Input: part model. Units: mm. Frame: model coordinates. Face numbers are marked on the shaded views. A direction names the side the tool comes from. Give positions to 0.01 mm unless a question says otherwise; leave off trailing zeros. Loops run counter-clockwise (first coordinate to the right, second up) from the corner with the lowest first, then second, coordinate; pieces in that order, holes last. Notation, with made-up numbers: (83, 77) -> (117, 77) arc R36 ccw to (117, 116) -> close; hole circle Ø8 at (22.25, 42). An arc over 180 degrees is marked (long way). One line per question, with ' | ' between items.
from build123d import *

# Parameters (mm, degrees)
SZKIC1_R                    = 323.75
DODANIE_WYCI_GNI_CIE1_DEPTH = 381
ZAOKR_GLENIE1_R             = 50
SZKIC2_R                    = 6.5
SZKIC2_R_2                  = 30
WYTNIJ_WYCI_GNI_CIE1_DEPTH  = 596.641775734
SZKIC3_R                    = 250
WYTNIJ_WYCI_GNI_CIE2_DEPTH  = 50
WYTNIJ_WYCI_GNI_CIE3_START  = -200
SZKIC4_R                    = 250
WYTNIJ_WYCI_GNI_CIE3_DEPTH  = 200
WYTNIJ_WYCI_GNI_CIE4_DEPTH  = 200
WYTNIJ_WYCI_GNI_CIE5_START  = -80
SZKIC6_R                    = 250
SZKIC6_R_2                  = 85
WYTNIJ_WYCI_GNI_CIE5_DEPTH  = 80


with BuildPart() as part:
    # Szkic1 → Dodanie-wyciągnięcie1 (new body)
    with BuildSketch(Plane.XY):
        Circle(SZKIC1_R)
    extrude(amount=DODANIE_WYCI_GNI_CIE1_DEPTH)

    # Zaokrąglenie1
    zaokr_glenie1_edges = [part.edges().sort_by_distance(p)[0] for p in [
        (-323.75, 0, 0),
        (-323.75, 0, 381),
    ]]
    fillet(zaokr_glenie1_edges, radius=ZAOKR_GLENIE1_R)

    # Szkic2 → Wytnij-wyciągnięcie1 (cut, through all)
    with BuildSketch(Plane.XY.offset(381)):
        with Locations((-60, 0)):
            Circle(SZKIC2_R)
        with Locations((-18.541019662, 57.063390978)):
            Circle(SZKIC2_R)
        with Locations((48.541019662, 35.267115138)):
            Circle(SZKIC2_R)
        with Locations((48.541019662, -35.267115138)):
            Circle(SZKIC2_R)
        with Locations((-18.541019662, -57.063390978)):
            Circle(SZKIC2_R)
        Circle(SZKIC2_R_2)
    extrude(amount=-WYTNIJ_WYCI_GNI_CIE1_DEPTH, mode=Mode.SUBTRACT)

    # Szkic3 → Wytnij-wyciągnięcie2 (cut)
    with BuildSketch(Plane.XY.offset(381)):
        Circle(SZKIC3_R)
    extrude(amount=-WYTNIJ_WYCI_GNI_CIE2_DEPTH, mode=Mode.SUBTRACT)

    # Szkic4 → Wytnij-wyciągnięcie3 (cut)
    with BuildSketch(Plane(origin=(0, 0, 0), x_dir=(-1, 0, 0), z_dir=(0, 0, -1)).offset(WYTNIJ_WYCI_GNI_CIE3_START)):
        with Locations(Location((0, 0, 0), (0, 0, 180))):
            Circle(SZKIC4_R)
    extrude(amount=WYTNIJ_WYCI_GNI_CIE3_DEPTH, mode=Mode.SUBTRACT)

    # Szkic5 → Wytnij-wyciągnięcie4 (cut)
    with BuildSketch(Plane.XY.offset(331)):
        Polygon((-96.155840105, 0), (-149.925673453, 63.746040452), (-231.191444309, 44.19337378), (-220.558452121, 0), (-96.155840105, -44.404647078), align=None)
        Polygon((-102.20240394, 27.791849476), (-73.659646986, 61.807782618), (-73.87456406, 145.202665329), (-148.695968113, 182.461084274), (-168.95757663, 141.772240235), align=None)
        Polygon((-60.427327118, 86.984230788), (-16.697286406, 94.695016833), (36.743274881, 158.71734935), (3.376004134, 235.353225607), (-38.29957328, 217.207673641), align=None)
        Polygon((9.622367637, 105.475723792), (48.077920052, 83.273400253), (130.168527149, 97.966421664), (153.868306527, 178.120977019), (110.279226061, 191.009222556), align=None)
        Polygon((75.169649634, 74.613953402), (90.356933392, 32.887234214), (162.686478902, -8.624083495), (232.36391824, 37.543943689), (207.25714991, 75.435433406), align=None)
        Polygon((105.54421715, 8.839484973), (90.356933392, -32.887234214), (119.081619118, -111.17928414), (202.133870171, -120.600318147), (207.25714991, -75.435433406), align=None)
        Polygon((86.533472468, -61.071076714), (48.077920052, -83.273400253), (19.757146304, -161.712462116), (77.323137782, -222.314350799), (110.279226061, -191.009222556), align=None)
        Polygon((27.032754306, -102.405802878), (-16.697286406, -94.695016833), (-88.811914842, -136.578581834), (-83.667950127, -220.005027963), (-38.29957328, -217.207673641), align=None)
        Polygon((-45.116890032, -95.823715761), (-73.659646986, -61.807782618), (-155.824893999, -47.53806521), (-205.509874305, -114.75290746), (-168.95757663, -141.772240235), align=None)
    extrude(amount=-WYTNIJ_WYCI_GNI_CIE4_DEPTH, mode=Mode.SUBTRACT)

    # Szkic6 → Wytnij-wyciągnięcie5 (cut)
    with BuildSketch(Plane(origin=(0, 0, 200), x_dir=(-1, 0, 0), z_dir=(0, 0, -1)).offset(WYTNIJ_WYCI_GNI_CIE5_START)):
        with Locations(Location((0, 0, 0), (0, 0, 180))):
            Circle(SZKIC6_R)
        Circle(SZKIC6_R_2, mode=Mode.SUBTRACT)
    extrude(amount=WYTNIJ_WYCI_GNI_CIE5_DEPTH, mode=Mode.SUBTRACT)


solid = part.part
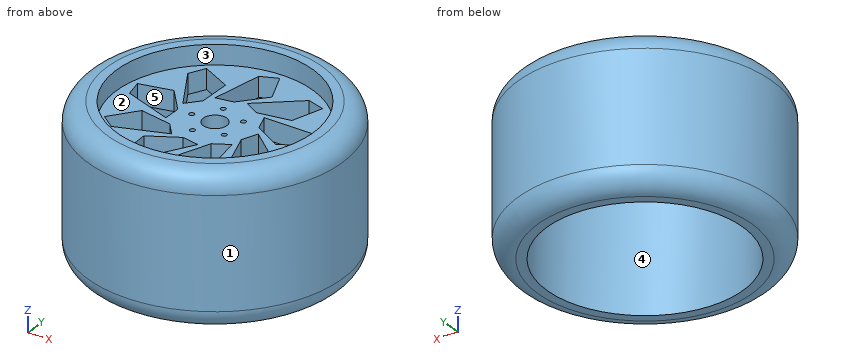
1. Pull-direction query (Y, two-part tool) for the marked faces 1 and 2; classes: pulls with the +Y half, pulls with the -Y half, needs draft (parallel to the pull), parting line crosses it, or undercut.
Determined:
face 1: parting line crosses it | face 2: undercut
2. Section query A-A (z = 244). Count the separate pieces of the cut face and the enclosed holes in it, then the cut area to 3 significant figures.
Determined:
separate pieces: 2 | enclosed holes: 7 | area: 152,000 mm2
3. Section query B-B (z = 141.5). Output: boundary loops of the cut face in (x, y).
Determined:
outline: circle Ø647.5 at (0, 0); hole circle Ø500 at (0, 0)
4. Ray query, line 1 along Y through (x, z) = (0, 237.5); line 2 along Y through (x, z) = (-48.5, 279.5); line 3 along Y through (x, z) = (0, 183). Return the intervals inside material, ascending. Write a range as from..to.
Determined:
line 1: y = -323.75..-250, -85..-30, 30..85, 250..323.75 | line 2: y = -320.1..-245.25, -69.81..69.81, 245.25..320.1 | line 3: y = -323.75..-250, 250..323.75
5. Reachability of the marked faces 3, 4 and 5 from +Z, -Z, +X, -X, +Y, -Y: full face, straight path, thin tool, end or side. Return the list, or none.
Determined:
face 3: +Z | face 4: -Z | face 5: +Z, -Z
6. Pin query (flat end, axial travel): P1, Ø10, axis at x = 168, z = 153.5, coming from the -Y side; P2, Ø1.5, axis at x = 236, y = -50, coming from the +Z side; P3, Ø5, axis at x = 42, y = -74.5, coming from the -Z side. Return the tip coordinate at first contact, or that it passes through.
Determined:
P1: stops at y = -279.72 | P2: stops at z = 331 | P3: stops at z = 200
